from build123d import *

# Parameters (mm, degrees)
SKETCH1_R            = 3
BOSS_EXTRUDE1_DEPTH  = 3.175
BOSS_EXTRUDE2_DEPTH  = 8.5
SKETCH3_R            = 7
BOSS_EXTRUDE3_DEPTH  = 3.175
SKETCH4_W            = 3.171981578
SKETCH4_H            = 25.4
BOSS_EXTRUDE4_DEPTH  = 42.45
SKETCH5_R            = 5
SKETCH5_R_2          = 3
BOSS_EXTRUDE5_DEPTH  = 5
CHAMFER2_SIZE        = 7.5
SKETCH7_W            = 25.4
SKETCH7_H            = 3.175
BOSS_EXTRUDE6_DEPTH  = 5.5
SKETCH9_W            = 25.4
SKETCH9_H            = 3.175
BOSS_EXTRUDE7_DEPTH  = 10
BOSS_EXTRUDE8_DEPTH  = 31
BOSS_EXTRUDE11_DEPTH = 3.175


with BuildPart() as part:
    # Sketch1 → Boss-Extrude1 (new body)
    with BuildSketch(Plane(origin=(0, 0, 0), x_dir=(0, 0, -1), z_dir=(1, 0, 0))):
        Polygon((-12.7, 12.7), (-12.7, 0), (-12.7, -13.638521551), (12.7, -13.638521551), (12.7, 0), (12.7, 12.7), align=None)
        Circle(SKETCH1_R, mode=Mode.SUBTRACT)
    extrude(amount=BOSS_EXTRUDE1_DEPTH)

    # Sketch2 → Boss-Extrude2 (add)
    with BuildSketch(Plane.ZY):
        Polygon((-10.7, -11.638521551), (-10.7, -13.638521551), (-12.7, -13.638521551), (-12.7, 12.7), (12.7, 12.7), (12.7, -13.638521551), (10.7, -13.638521551), (10.7, -11.638521551), (10.7, 10.7), (-10.7, 10.7), align=None)
    extrude(amount=BOSS_EXTRUDE2_DEPTH)

    # Sketch3 → Boss-Extrude3 (add)
    with BuildSketch(Plane.ZY.offset(8.5)):
        Polygon((-10.7, -13.638521551), (10.7, -13.638521551), (12.7, -13.638521551), (12.7, 12.7), (-12.7, 12.7), (-12.7, -13.638521551), align=None)
        Circle(SKETCH3_R, mode=Mode.SUBTRACT)
    extrude(amount=BOSS_EXTRUDE3_DEPTH)

    # Sketch4 → Boss-Extrude4 (add)
    with BuildSketch(Plane.XZ.offset(13.638521551)):
        with Locations((-10.089009211, 0)):
            Rectangle(SKETCH4_W, SKETCH4_H)
    extrude(amount=BOSS_EXTRUDE4_DEPTH)

    # Sketch5 → Boss-Extrude5 (add)
    with BuildSketch(Plane(origin=(3.175, 0, 0), x_dir=(0, 0, -1), z_dir=(1, 0, 0))):
        Circle(SKETCH5_R)
        Circle(SKETCH5_R_2, mode=Mode.SUBTRACT)
    extrude(amount=BOSS_EXTRUDE5_DEPTH)

    # Chamfer2
    chamfer2_edges = [part.edges().sort_by_distance(p)[0] for p in [
        (-4.25, 12.7, 12.7),
        (-4.25, 12.7, -12.7),
        (-4.25, 10.7, -10.7),
        (-4.25, 10.7, 10.7),
    ]]
    chamfer(chamfer2_edges, length=CHAMFER2_SIZE)

    # Sketch7 → Boss-Extrude6 (add)
    with BuildSketch(Plane(origin=(-8.503018422, 0, 0), x_dir=(0, 0, -1), z_dir=(1, 0, 0))):
        with Locations((0, -18.226021551)):
            Rectangle(SKETCH7_W, SKETCH7_H)
    extrude(amount=BOSS_EXTRUDE6_DEPTH)

    # Sketch9 → Boss-Extrude7 (add)
    with BuildSketch(Plane(origin=(-8.503018422, 0, 0), x_dir=(0, 0, -1), z_dir=(1, 0, 0))):
        with Locations((0, -54.501021551)):
            Rectangle(SKETCH9_W, SKETCH9_H)
    extrude(amount=BOSS_EXTRUDE7_DEPTH)

    # Sketch10 → Boss-Extrude8 (add)
    with BuildSketch(Plane(origin=(3.175, 0, 0), x_dir=(0, 0, -1), z_dir=(1, 0, 0))):
        Polygon((5.2, 12.7), (-5.2, 12.7), (-12.7, 5.2), (-12.7, -13.638521551), (-10.7, -13.638521551), (-10.7, -11.638521551), (-10.7, 4.371572875), (-4.371572875, 10.7), (4.371572875, 10.7), (10.7, 4.371572875), (10.7, -11.638521551), (10.7, -13.638521551), (12.7, -13.638521551), (12.7, 5.2), align=None)
    extrude(amount=BOSS_EXTRUDE8_DEPTH)

    # Sketch12 → Boss-Extrude11 (add)
    with BuildSketch(Plane.XY.offset(12.7)):
        Polygon((-11.675, -52.913521551), (-11.675, -56.088521551), (1.496981578, -56.088521551), (1.496981578, -52.913521551), (37.215, -52.913521551), (37.215, -16.638521551), (-11.675, -16.638521551), align=None)
    extrude(amount=BOSS_EXTRUDE11_DEPTH)


solid = part.part
Check sheet for the modelled part. Datum: model origin and axes. Units: mm. A direction names the side the tool comes from. Give positions to 0.01 mm unless a question says otherwise; leave off trailing zeros. Loops run counter-clockwise (first coordinate to the right, second up) from the corner with the lowest first, then second, coordinate; pieces in that order, holes last. Notation, with made-up numbers: M 55.25,-38 L 63.25,-38 A29 ccw 63.25,-4 Z; hole C 20.5,-8 d7. An arc over 180 degrees is marked long. Return JSON: item names as keys, results as strings. Group by question number.
1. Thickness scan on L1, parallel to Y at x = 6, z = 0; L2, parallel to Y at x = -10.4, z = 0; L3, parallel to Y at x = 2, z = 0. Record the ranges inside material, lowest first.
2. Cross-section at D-D on y = -9. Record the boundary of the cut face in (x, z) (3 decimals).
3. Cross-section at B-B on x = 10. Record the boundary of the cut face in (y, z) (3 decimals).
4. Cross-section at C-C on z = 0. State how many separate pieces and enclosed holes the cut face has, plus the area to 3 significant figures.
5. Mould release check, pull along X, two halves, no side actions. Record for faces 5 (the flat face through (0, -4, 0)), 6 (the flat face through (34.175, 11, 0)), 7 (the cylindrical face through (4, 0, 3)), 8 (the flat face through (-4, 10.7, 0)): released by +X, released by -X, zero draft, split by the parting line, or undercut.
6. Go/stop test with flat-tipped pins: pin 1 (8.5 mm diameter, centred on y = 0, z = 0, fed in from +X) (3 decimals); pin 2 (3 mm diameter, centred on x = -0.5, y = -4.5, fed in from +Z); pin 3 (10 mm diameter, centred on x = 25.5, y = -44.5, fed in from -Z); pin 4 (8 mm diameter, centred on x = 3, z = 12, fed in from -Y). Record where each tip stops, or that it passes through.
7. Cross-section at A-A on y = 0. Record the boundary of the cut face in (x, z) (3 decimals), plus the area to 3 significant figures.
8. Tool access check on faces 1 (the flat face through (1.497, -55, 1)), 2 (the flat face through (-8.503, -36, 0)), 3 (the cylindrical face through (-10.065, -2.681, 6.466)), 4 (the flat face through (-8.503, -15, 0)). Record the directions out of +Z, -Z, +X, -X, +Y, -Y that give a thin tool (end or side, any length) a straight path to the whole face; none if there is none.
Return value:
{
 "1": {"L1": "-5 to -3, 3 to 5, 10.7 to 12.7", "L2": "-56.09 to -7, 7 to 12.7", "L3": "-13.64 to -3, 3 to 12.7"},
 "2": {"outline": "M -11.675,-12.7 L 34.175,-12.7 L 34.175,-10.7 L 3.175,-10.7 L 3.175,10.7 L 34.175,10.7 L 34.175,12.7 L -11.675,12.7 Z; hole M -8.5,-10.7 L 0,-10.7 L 0,10.7 L -8.5,10.7 Z"},
 "3": {"outline": "M -52.914,12.7 L -16.639,12.7 L -16.639,15.875 L -52.914,15.875 Z; M -13.639,-12.7 L 5.2,-12.7 L 12.7,-5.2 L 12.7,5.2 L 5.2,12.7 L -13.639,12.7 L -13.639,10.7 L 4.372,10.7 L 10.7,4.372 L 10.7,-4.372 L 4.372,-10.7 L -13.639,-10.7 Z"},
 "4": {"separate pieces": "3", "enclosed holes": "0", "area": "387 mm^2"},
 "5": {"face 5": "undercut", "face 6": "released by +X", "face 7": "zero draft", "face 8": "undercut"},
 "6": {"pin 1": "x = 8.175", "pin 2": "z = 12.7", "pin 3": "z = 12.7", "pin 4": "y = -56.09"},
 "7": {"outline": "M -11.675,-12.7 L 34.175,-12.7 L 34.175,-10.7 L 3.175,-10.7 L 3.175,-5 L 8.175,-5 L 8.175,-3 L 0,-3 L 0,-10.7 L -8.5,-10.7 L -8.5,-7 L -11.675,-7 Z; M -11.675,7 L -8.5,7 L -8.5,10.7 L 0,10.7 L 0,3 L 8.175,3 L 8.175,5 L 3.175,5 L 3.175,10.7 L 34.175,10.7 L 34.175,12.7 L -11.675,12.7 Z", "area": "276 mm^2"},
 "8": {"face 1": "+Z, -Z, +X, -Y", "face 2": "-Z, +X", "face 3": "-X", "face 4": "+Z, -Z, +X"}
}
